```python
from build123d import *

# Parameters (mm, degrees)
F0_R     = 1.7
F1_DEPTH = 1.5
F2_R     = 1.7
F3_DEPTH = 1.5
F5_DEPTH = 8
F6_R     = 19
F6_R_2   = 1.5
F7_DEPTH = 3.001


with BuildPart() as f1:
    # F0 (on Top) → F1 (new body)
    with BuildSketch(Plane.XY):
        Polygon((3.421573, -3.5), (-3.421573, -3.5), (-9.078427, -3.5), (-20, -3.5), (-20, -6.5), (20, -6.5), (20, -3.5), (9.078427, -3.5), align=None)
        with BuildLine():
            Line((-9.078427, -3.5), (-3.421573, -3.5))
            ThreePointArc((-3.421573, -3.5), (-1.752972, 0.163508), (-3.683219, 3.696165))
            ThreePointArc((-3.683219, 3.696165), (-9.85046, 2.699387), (-9.078427, -3.5))
        make_face()
        with Locations((-6.25, 0)):
            Circle(F0_R, mode=Mode.SUBTRACT)
        with BuildLine():
            ThreePointArc((-3.683219, 3.696165), (-1.752972, 0.163508), (-3.421573, -3.5))
            Line((-3.421573, -3.5), (3.421573, -3.5))
            ThreePointArc((3.421573, -3.5), (1.755629, -0.225008), (3.086142, 3.2))
            Line((3.086142, 3.2), (2.838445, 3.2))
            ThreePointArc((2.838445, 3.2), (-0.489853, 2.561303), (-3.683219, 3.696165))
        make_face()
        with BuildLine():
            ThreePointArc((3.086142, 3.2), (1.755629, -0.225008), (3.421573, -3.5))
            Line((3.421573, -3.5), (9.078427, -3.5))
            ThreePointArc((9.078427, -3.5), (10.744371, -0.225008), (9.413858, 3.2))
            Line((9.413858, 3.2), (3.086142, 3.2))
        make_face()
        with Locations((6.25, 0)):
            Circle(F0_R, mode=Mode.SUBTRACT)
        with BuildLine():
            ThreePointArc((3.683219, 3.696165), (3.270255, 3.432038), (2.838445, 3.2))
            Line((2.838445, 3.2), (3.086142, 3.2))
            Line((3.086142, 3.2), (9.413858, 3.2))
            ThreePointArc((9.413858, 3.2), (6.638163, 4.483228), (3.683219, 3.696165))
        make_face()
    extrude(amount=F1_DEPTH)

    # F2 (on face) → F3 (join)
    with BuildSketch(Plane.XY.offset(1.5)):
        with BuildLine():
            Line((-9.078427, -3.5), (-3.421573, -3.5))
            ThreePointArc((-3.421573, -3.5), (-1.752972, 0.163508), (-3.683219, 3.696165))
            ThreePointArc((-3.683219, 3.696165), (-9.85046, 2.699387), (-9.078427, -3.5))
        make_face()
        with Locations((-6.25, 0)):
            Circle(F2_R, mode=Mode.SUBTRACT)
        with BuildLine():
            ThreePointArc((-3.683219, 3.696165), (-1.752972, 0.163508), (-3.421573, -3.5))
            Line((-3.421573, -3.5), (3.421573, -3.5))
            ThreePointArc((3.421573, -3.5), (1.755629, -0.225008), (3.086142, 3.2))
            Line((3.086142, 3.2), (2.838445, 3.2))
            ThreePointArc((2.838445, 3.2), (-0.489853, 2.561303), (-3.683219, 3.696165))
        make_face()
        with BuildLine():
            ThreePointArc((3.086142, 3.2), (1.755629, -0.225008), (3.421573, -3.5))
            Line((3.421573, -3.5), (9.078427, -3.5))
            ThreePointArc((9.078427, -3.5), (10.744371, -0.225008), (9.413858, 3.2))
            Line((9.413858, 3.2), (3.086142, 3.2))
        make_face()
        with Locations((6.25, 0)):
            Circle(F2_R, mode=Mode.SUBTRACT)
        Polygon((3.421573, -3.5), (-3.421573, -3.5), (-9.078427, -3.5), (-20, -3.5), (-20, -6.5), (20, -6.5), (20, -3.5), (9.078427, -3.5), align=None)
    extrude(amount=F3_DEPTH)

    # F4 (on face) → F5 (join)
    with BuildSketch(Plane.XY.offset(3)):
        Polygon((3.421573, -3.5), (-3.421573, -3.5), (-9.078427, -3.5), (-20, -3.5), (-20, -6.5), (20, -6.5), (20, -3.5), (9.078427, -3.5), align=None)
    extrude(amount=F5_DEPTH)

    # F6 (on face) → F7 (cut, through all)
    with BuildSketch(Plane(origin=(0, -3.5, 0), x_dir=(-1, 0, 0), z_dir=(0, 1, 0))):
        with Locations((0, 23)):
            Circle(F6_R)
        with Locations((-16, 7)):
            Circle(F6_R_2)
        with Locations((16, 7)):
            Circle(F6_R_2)
    extrude(amount=-F7_DEPTH, mode=Mode.SUBTRACT)


solid = f1.part
```
Check sheet for the modelled part. Datum: model origin and axes. Units: mm. A direction names the side the tool comes from. Give positions to 0.01 mm unless a question says otherwise; leave off trailing zeros. Write each loop counter-clockwise with the first axis right and the second up, starting at its lowest first coordinate (ties: lowest second). Pieces come first, ordered by that corner, then holes.
Item 1: Cross-section at C-C (y = 0). Enter the section's corners in (x, z), and give its area (3 significant figures).
Item 2: Access from +Z, -Z, +X, -X, +Y, -Y to the whole of each face (thin tool, end or side, straight path). Record for faces 4 (the face through (0, 0, 3)), 5 (the face through (6, 3.2, 2)), 6 (the face through (3.28, 3.44, 0.74)).
Item 3: Cross-section at B-B (x = -5.5). Enter the section's corners in (y, z), and give its area (3 significant figures).
Item 4: Cross-section at D-D (z = 9.25). Enter the section's corners in (x, y).
Item 5: Draft check along X on faces 1 (the face through (-6.62, -1.66, 1.48)), 2 (the face through (6, 4, 1.5)), 3 (the face through (-20, -5, 5)). Enter one of: released by +X, released by -X, zero draft, split by the parting line, or undercut.
Item 6: Scan lines: L1, parallel to Y at x = 6.25, z = 2.1; L2, parallel to Y at x = -6.25, z = 1.35; L3, parallel to X at y = -0.5, z = 2.5. Record each from-to range of solid material in increasing order.
Item 7: Gauge pin test, flat ends, axial feed: pin 1 (1.2 mm diameter, centred on x = 7, z = 2, fed in from +Y); pin 2 (1 mm diameter, centred on x = -7, y = 1.5, fed in from +Z). Record the tip position at first contact, or that the pin passes through.
Item 8: Cross-section at A-A (y = -5.5). Enter the section's corners in (x, z).
Report:
1. outline: (-10.75, 0) - (-7.95, 0) - (-7.95, 3) - (-10.75, 3) - close; (-4.55, 0) - (4.55, 0) - (4.55, 3) - (-4.55, 3) - close; (7.95, 0) - (10.75, 0) - (10.75, 3) - (7.95, 3) - close
1. area: 44.1 mm2
2. face 4: +Z, +X, -X, +Y
2. face 5: +Z, +X, +Y
2. face 6: +Z, -Z, +Y
3. outline: (-6.5, 0) - (-1.53, 0) - (-1.53, 3) - (-3.5, 3) - (-3.5, 4.81) - (-6.5, 4.81) - close; (1.53, 0) - (4.44, 0) - (4.44, 3) - (1.53, 3) - close
3. area: 29.1 mm2
4. outline: (-20, -6.5) - (-13.11, -6.5) - (-13.11, -3.5) - (-20, -3.5) - close; (13.11, -6.5) - (20, -6.5) - (20, -3.5) - (13.11, -3.5) - close
5. face 1: undercut
5. face 2: zero draft
5. face 3: released by -X
6. L1: y = -6.5 to -1.7, 1.7 to 3.2
6. L2: y = -6.5 to -1.7, 1.7 to 4.5
6. L3: x = -10.72 to -7.87, -4.63 to 4.63, 7.87 to 10.72
7. pin 1: stops at y = 4.48
7. pin 2: stops at z = 3
8. outline: (-20, 0) - (20, 0) - (20, 11) - (14.73, 11) arc R19 cw to (-14.73, 11) - (-20, 11) - close; hole circle Ø3 at (-16, 7); hole circle Ø3 at (16, 7)
